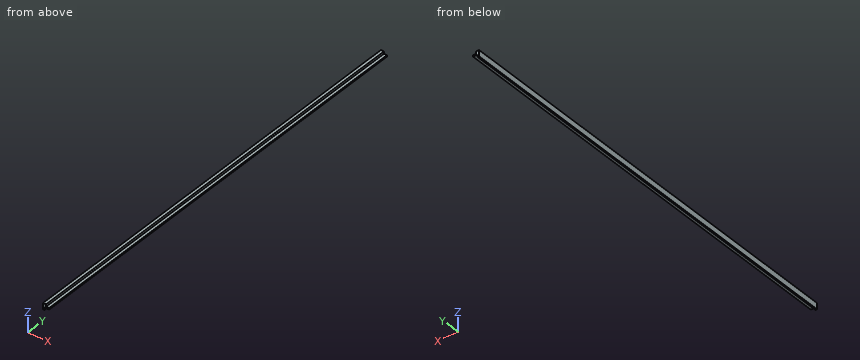
```python
from build123d import *

# Parameters (mm, degrees)
F0_W     = 12.7
F0_H     = 12.7
F1_DEPTH = 914.4
F2_W     = 9.525
F2_H     = 4.7625
F3_DEPTH = 914.401
F4_W     = 6.35
F4_H     = 4.7625
F5_DEPTH = 914.401


with BuildPart() as f1:
    # F0 (on Front) → F1 (new body)
    with BuildSketch(Plane.XZ):
        with Locations((6.35, 6.35)):
            Rectangle(F0_W, F0_H)
    extrude(amount=F1_DEPTH)

    # F2 (on Front) → F3 (cut, through all)
    with BuildSketch(Plane.XZ):
        with Locations((7.9375, 2.38125)):
            Rectangle(F2_W, F2_H)
    extrude(amount=F3_DEPTH, mode=Mode.SUBTRACT)

    # F4 (on Front) → F5 (cut, through all)
    with BuildSketch(Plane.XZ):
        with Locations((9.525, 10.31875)):
            Rectangle(F4_W, F4_H)
    extrude(amount=F5_DEPTH, mode=Mode.SUBTRACT)


solid = f1.part
```
Geometry check sheet. Reference: the model listing, model coordinates, mm. Round coordinates to 2 decimals unless told otherwise and drop trailing zeros. Write each loop counter-clockwise with the first axis right and the second up, starting at its lowest first coordinate (ties: lowest second). Pieces come first, ordered by that corner, then holes. Notation, with made-up numbers: (-28, 12) -> (9, 12) arc R22 cw to (9, 21) -> close; hole circle Ø7 at (-10.5, -13.5). An arc over 180 degrees is marked (long way). Put each result on its own line as item: value.
1) Cross-section at C-C, the plane z = 2.75. Enter the section's corners in (x, y) (3 decimals).
Recorded:
outline: (0, -914.4) -> (3.175, -914.4) -> (3.175, 0) -> (0, 0) -> close
2) Cross-section at B-B, the plane x = 8.5. Enter the section's corners in (y, z), plus the area to 3 significant figures.
Recorded:
outline: (-914.4, 4.76) -> (0, 4.76) -> (0, 7.94) -> (-914.4, 7.94) -> close
area: 2,900 mm2
3) Thickness scan on probe 1 along X at (y, z) = (-558, 9.5); probe 2 along Z at (x, y) = (11, -39.5); probe 3 along X at (y, z) = (-111, 4.25) (3 decimals). Record the ranges inside material, lowest first. Write a range as from..to.
Recorded:
probe 1: x = 0..6.35
probe 2: z = 4.76..7.94
probe 3: x = 0..3.175
4) Depth check by flat-ended pin: P1, Ø6, axis at x = 4.5, y = -699, coming from the -Z side; P2, Ø5, axis at y = -507, z = 11, coming from the +X side; P3, Ø1, axis at x = 10, y = -472.5, coming from the +Z side; P4, Ø5, axis at x = 6.5, y = -420, coming from the -Z side. Enter the tip coordinate at first touch or a pass-through.
Recorded:
P1: stops at z = 0
P2: stops at x = 6.35
P3: stops at z = 7.94
P4: stops at z = 4.76
